The listing builds one solid part. Answer for the finished solid, in the listing's coordinates (mm). A direction names the side the tool comes from. Round coordinates to 2 decimals unless told otherwise and drop trailing zeros. Order: outer loops, then holes, each group sorted by start corner. A loop starts at its lowest first (then second) coordinate and runs counter-clockwise, first axis right, second up. Notation, with made-up numbers: (-14, -21.5) -> (13, -21.5) arc R14 cw to (13, 5.5) -> close; hole circle Ø4 at (40.25, -16.5). An arc over 180 degrees is marked (long way). Answer in a Markdown table with one row per item. Add a question column.
```python
from build123d import *

# Parameters (mm, degrees)
SKETCH1_W           = 8
SKETCH1_H           = 7.9
BOSS_EXTRUDE1_DEPTH = 2.9
SKETCH2_W           = 8
SKETCH2_H           = 4.9
BOSS_EXTRUDE2_DEPTH = 6
SKETCH4_W           = 8
SKETCH4_H           = 2.8
BOSS_EXTRUDE3_DEPTH = 8


with BuildPart() as part:
    # Sketch1 → Boss-Extrude1 (new body)
    with BuildSketch(Plane(origin=(0, 0, 0), x_dir=(1, 0, 0), z_dir=(0, 1, 0))):
        with Locations((4, 3.95)):
            Rectangle(SKETCH1_W, SKETCH1_H)
    extrude(amount=BOSS_EXTRUDE1_DEPTH)

    # Sketch2 → Boss-Extrude2 (add)
    with BuildSketch(Plane(origin=(0, 2.9, 0), x_dir=(1, 0, 0), z_dir=(0, 1, 0))):
        with Locations((4, 3.95)):
            Rectangle(SKETCH2_W, SKETCH2_H)
    extrude(amount=BOSS_EXTRUDE2_DEPTH)

    # Sketch4 → Boss-Extrude3 (add, through all)
    with BuildSketch(Plane.ZY):
        with Locations((-3.95, 7.5)):
            Rectangle(SKETCH4_W, SKETCH4_H)
    extrude(amount=-BOSS_EXTRUDE3_DEPTH)

    # Sketch3 → Cut-Revolve2 (revolve, cut)
    with BuildSketch(Plane.ZY.offset(-4)):
        with BuildLine():
            Line((-3.95, 8.9), (-6.399489743, 8.9))
            ThreePointArc((-6.399489743, 8.9), (-5.886491673, 6.81886117), (-3.95, 5.9))
            Line((-3.95, 5.9), (-3.95, 8.9))
        make_face()
    revolve(axis=Axis((4, 8.9, -3.95), (0, -1, 0)), mode=Mode.SUBTRACT)


solid = part.part
```
Item 1: Flat-ended cylindrical pins translate along their axes: P1, Ø1, axis at x = 3, y = 5, coming from the +Z side; P2, Ø1.4, axis at x = 3, y = 1, coming from the -Z side; P3, Ø2.5, axis at x = 4.5, y = 0.5, coming from the +Z side. Find the tip coordinate at first contact, or state that the pin passes through.
Item 2: The part is cut by section B-B, the plane x = 0.75. Give the vertices of the cut face in (y, z), and give its area (3 significant figures).
Item 3: The part is cut by section D-D, the plane y = 4. Give the vertices of the cut face in (x, z).
Item 4: Find the intervals of material crossed by probe 1 along Y at (x, z) = (2.75, -0.75); probe 2 along Z at (x, y) = (2.25, 4.5); probe 3 along Z at (x, y) = (2.25, 1), in increasing order. Write a range as [from, to].
Item 5: A tool of negligible diameter and unlimited length cuts with its end or side. For faces 4 (the face through (4, 6.1, -1)), 5 (the face through (4, 7, 0.05)), 6 (the face through (4, 1, -7.9)), 7 (the face through (4, 1, 0)), 8 (the face through (4, 6.1, -7)), from which of +Z, -Z, +X, -X, +Y, -Y can it reach the whole face along a straight path? Write none if from no direction.
Item 6: For a pull along Y with two mould halves and no side action, classify faces 1 (the face through (2, 8.9, -6)), 2 (the face through (4, 2.9, -1)), 3 (the face through (4, 0, -4)) as released by +Y, released by -Y, zero draft, split by the parting line, or undercut.
Item 7: The part is cut by section A-A, the plane z = -1.25. Give the vertices of the cut face in (x, y), and give its area (3 significant figures).
Item 8: The part is cut by section C-C, the plane y = 6.75. Give the vertices of the cut face in (x, z).
Resolved:
| question | item | result |
|---|---|---|
| 1 | P1 | z = -1.5 |
| 1 | P2 | z = -7.9 |
| 1 | P3 | z = 0 |
| 2 | outline | (0, -7.9) -> (2.9, -7.9) -> (2.9, -6.4) -> (6.1, -6.4) -> (6.1, -7.95) -> (8.9, -7.95) -> (8.9, 0.05) -> (6.1, 0.05) -> (6.1, -1.5) -> (2.9, -1.5) -> (2.9, 0) -> (0, 0) -> close |
| 2 | area | 61.0 mm2 |
| 3 | outline | (0, -6.4) -> (8, -6.4) -> (8, -1.5) -> (0, -1.5) -> close |
| 4 | probe 1 | [0, 2.9], [6.1, 8.9] |
| 4 | probe 2 | [-6.4, -1.5] |
| 4 | probe 3 | [-7.9, 0] |
| 5 | face 4 | +Z, +X, -X |
| 5 | face 5 | +Z, +X, -X, +Y, -Y |
| 5 | face 6 | -Z, +X, -X, -Y |
| 5 | face 7 | +Z, +X, -X, -Y |
| 5 | face 8 | -Z, +X, -X |
| 6 | face 1 | released by +Y |
| 6 | face 2 | undercut |
| 6 | face 3 | released by -Y |
| 7 | outline | (0, 0) -> (8, 0) -> (8, 2.9) -> (0, 2.9) -> close; (0, 6.1) -> (8, 6.1) -> (8, 8.9) -> (0, 8.9) -> close |
| 7 | area | 45.6 mm2 |
| 8 | outline | (0, -7.95) -> (8, -7.95) -> (8, 0.05) -> (0, 0.05) -> close; hole circle Ø3.76 at (4, -3.95) |
